Could you check a few things on this model? Use its own coordinates, in mm. A direction names the side the tool comes from. Coordinates: 2 decimals unless noted, no trailing zeros. Loops run counter-clockwise (first coordinate to the right, second up) from the corner with the lowest first, then second, coordinate; pieces in that order, holes last. Notation, with made-up numbers: (73.25, 56) -> (124.25, 56) arc R17 ccw to (124.25, 87) -> close; hole circle Ø3 at (54, 29.5). An arc over 180 degrees is marked (long way). One line per question, with ' | ' between items.
```python
from build123d import *

# Parameters (mm, degrees)
SKETCH1_R           = 2.75
BOSS_EXTRUDE1_DEPTH = 2
FILLET1_R           = 0.4
SKETCH2_W           = 7.85101285
SKETCH2_H           = 1
CUT_EXTRUDE1_DEPTH  = 1
SKETCH3_R           = 1.5
BOSS_EXTRUDE2_DEPTH = 30


with BuildPart() as part:
    # Sketch1 → Boss-Extrude1 (new body)
    with BuildSketch(Plane.XY):
        Circle(SKETCH1_R)
    extrude(amount=BOSS_EXTRUDE1_DEPTH)

    # Fillet1
    fillet1_edges = [part.edges().sort_by_distance(p)[0] for p in [
        (-2.75, 0, 2),
    ]]
    fillet(fillet1_edges, radius=FILLET1_R)

    # Sketch2 → Cut-Extrude1 (cut)
    with BuildSketch(Plane.XY.offset(2)):
        Rectangle(SKETCH2_W, SKETCH2_H)
    extrude(amount=-CUT_EXTRUDE1_DEPTH, mode=Mode.SUBTRACT)

    # Sketch3 → Boss-Extrude2 (add)
    with BuildSketch(Plane(origin=(0, 0, 0), x_dir=(-1, 0, 0), z_dir=(0, 0, -1))):
        Circle(SKETCH3_R)
    extrude(amount=BOSS_EXTRUDE2_DEPTH)


solid = part.part
```
Q1. For pin 1 (0.8 mm diameter, centred on x = 0, y = 0, fed in from +Z); pin 2 (3 mm diameter, centred on x = 1.5, y = -0.5, fed in from -Z); pin 3 (1 mm diameter, centred on y = -1.5, z = -22, fed in from -X); pin 4 (0.8 mm diameter, centred on x = 1, z = 1.5, fed in from +Y), each with a flat end and sliding along its axis, tell me the tip position at first contact or that it passes through.
Values follow:
pin 1: stops at z = 1 | pin 2: stops at z = -30 | pin 3: stops at x = -1.12 | pin 4: stops at y = 2.68
Q2. Imagine slicing it at B-B on x = 0. Write out the boundary of the cut face in (y, z), plus the area to 3 significant figures.
Values follow:
outline: (-2.75, 0) -> (-1.5, 0) -> (-1.5, -30) -> (1.5, -30) -> (1.5, 0) -> (2.75, 0) -> (2.75, 1.6) arc R0.4 ccw to (2.35, 2) -> (0.5, 2) -> (0.5, 1) -> (-0.5, 1) -> (-0.5, 2) -> (-2.35, 2) arc R0.4 ccw to (-2.75, 1.6) -> close | area: 99.9 mm2
Q3. For faces 1 (the face through (1.2, -1.2, 0)), 2 (the face through (2.54, -1.05, 0.79)), 3 (the face through (0, 0.5, 1.5)), which set-ups out of +Z, -Z, +X, -X, +Y, -Y let a thin tool reach every point of the face, with its end or its side?
Values follow:
face 1: -Z | face 2: +Z, -Z | face 3: +Z, +X, -X
Q4. Imagine slicing it at C-C on z = -17.5. Write out the boundary of the cut face in (x, y), plus the area to 3 significant figures.
Values follow:
outline: circle Ø3 at (0, 0) | area: 7.07 mm2
Q5. We'd pull the mould along Y, two halves only. Please class faces 4 (the face through (0, 1, 2)), 5 (the face through (0, -0.5, 1.5)), 6 (the face through (1.5, 0.07, -14.79)): released by +Y, released by -Y, zero draft, split by the parting line, or undercut.
Values follow:
face 4: zero draft | face 5: undercut | face 6: split by the parting line
Q6. Imagine slicing it at A-A on y = 0. Write out the boundary of the cut face in (x, z).
Values follow:
outline: (-2.75, 0) -> (-1.5, 0) -> (-1.5, -30) -> (1.5, -30) -> (1.5, 0) -> (2.75, 0) -> (2.75, 1) -> (-2.75, 1) -> close
Q7. Please list where these lines run through material, in increasing order: L1, parallel to Z at x = -1.1, y = -1.45; L2, parallel to X at y = 0.7, z = -28; L3, parallel to Y at x = 0.8, z = -24.5. Write a range as [from, to].
Values follow:
L1: z = [0, 2] | L2: x = [-1.33, 1.33] | L3: y = [-1.27, 1.27]
